Geometry: final body of the model. Coordinates: model frame, mm. Round coordinates to 2 decimals unless told otherwise and drop trailing zeros. Loops run counter-clockwise (first coordinate to the right, second up) from the corner with the lowest first, then second, coordinate; pieces in that order, holes last. Notation, with made-up numbers: (-34.75, -30.5) -> (-14.75, -30.5) arc R15 ccw to (-14.75, -22.5) -> close; hole circle Ø3 at (15, -20). An arc over 180 degrees is marked (long way). Answer in a Markdown table with one row per item.
Autodesk Inventor part; units mm, degrees
ref_plane "YZ Plane" through (0, 0, 0) normal (1, 0, 0) x (0, 1, 0)
ref_plane "XZ Plane" through (0, 0, 0) normal (0, 1, 0) x (-1, 0, 0)
ref_plane "XY Plane" through (0, 0, 0) normal (0, 0, 1) x (1, 0, 0)
sketch "Sketch1" plane through (0, 0, 0) normal (0, 0, 1) x (1, 0, 0)
  line L0 (-75, -15.375) -> (-69, -15.375)
  line L1 (-69, -46.125) -> (-75, -46.125)
  line L2 (-69, 46.125) -> (-75, 46.125)
  line L3 (-75, 15.375) -> (-69, 15.375)
  line L4 (-69, 46.125) -> (-69, 69)
  line L5 (-75, 46.125) -> (-75, 15.375)
  line L6 (-69, 15.375) -> (-69, -15.375)
  line L7 (-75, -15.375) -> (-75, -46.125)
  line L8 (-69, -46.125) -> (-69, -69)
  line L9 (0, 0) -> (0, 15.375)
  line L10 (0, 0) -> (0, -46.125)
  line L11 (69, 15.375) -> (69, -15.375)
  line L12 (75, 15.375) -> (69, 15.375)
  line L13 (75, 46.125) -> (75, 15.375)
  line L14 (69, 46.125) -> (75, 46.125)
  line L15 (69, 46.125) -> (69, 69)
  line L16 (75, -15.375) -> (69, -15.375)
  line L17 (75, -15.375) -> (75, -46.125)
  line L18 (69, -46.125) -> (75, -46.125)
  line L19 (69, -46.125) -> (69, -69)
  line L20 (0, 0) -> (92.4518, 92.4518)
  line L21 (0, 0) -> (102.0745, -102.0745)
  line L22 (-15.375, 75) -> (-15.375, 69)
  line L23 (-46.125, 69) -> (-46.125, 75)
  line L24 (-15.375, 75) -> (-46.125, 75)
  line L25 (-46.125, 69) -> (-69, 69)
  line L26 (15.375, 69) -> (-15.375, 69)
  line L27 (15.375, 75) -> (15.375, 69)
  line L28 (46.125, 75) -> (15.375, 75)
  line L29 (46.125, 69) -> (46.125, 75)
  line L30 (46.125, 69) -> (69, 69)
  line L31 (46.125, -69) -> (46.125, -75)
  line L32 (46.125, -75) -> (15.375, -75)
  line L33 (46.125, -69) -> (69, -69)
  line L34 (-15.375, -75) -> (-15.375, -69)
  line L35 (15.375, -75) -> (15.375, -69)
  line L36 (15.375, -69) -> (-15.375, -69)
  line L37 (-15.375, -75) -> (-46.125, -75)
  line L38 (-46.125, -69) -> (-46.125, -75)
  line L39 (-46.125, -69) -> (-69, -69)
  line L40 (0, 0) -> (-28, 0)
  circle A0 centre (-28, 0) radius 20
  point P0 (0, 0)
  point P1 (0, 0)
  point P2 (-69, -75)
  point P3 (-69, 75)
  point P4 (69, -75)
  point P5 (69, 75)
  dimension "d1" = 28
  dimension "d2" = 40
extrude "Extrusion1" add sketch "Sketch1" along normal blind 6
properties part number "Top"
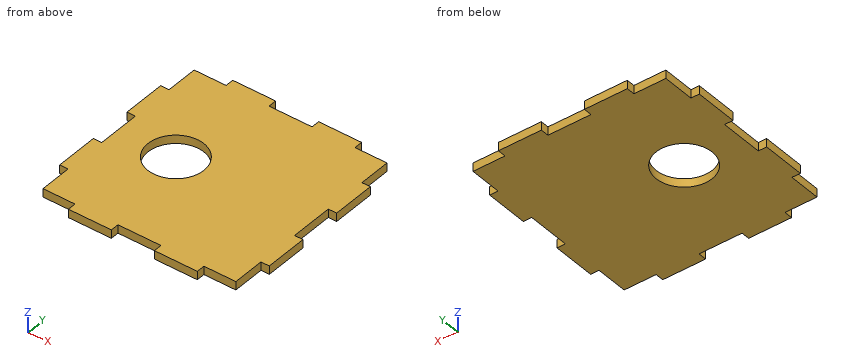
Item 1: Section query A-A, the plane x = -28. Output: boundary loops of the cut face in (y, z), and give its area (3 significant figures).
Ans:
| item | result |
|---|---|
| outline | (-75, 0) -> (-20, 0) -> (-20, 6) -> (-75, 6) -> close; (20, 0) -> (75, 0) -> (75, 6) -> (20, 6) -> close |
| area | 660 mm2 |
Item 2: Section query B-B, the plane y = 0. Output: boundary loops of the cut face in (x, z), and give its area (3 significant figures).
Ans:
| item | result |
|---|---|
| outline | (-69, 0) -> (-48, 0) -> (-48, 6) -> (-69, 6) -> close; (-8, 0) -> (69, 0) -> (69, 6) -> (-8, 6) -> close |
| area | 588 mm2 |
Item 3: First-contact query: P1, Ø1.8, axis at y = -72.5, z = 4.5, coming from the +X side (3 decimals); P2, Ø3, axis at y = -54, z = 3.5, coming from the -X side; P3, Ø1.8, axis at x = -71.5, z = 3, coming from the +Y side (3 decimals). Flat tips, straight axial feed; report the tip coordinate or a pass-through.
Ans:
| item | result |
|---|---|
| P1 | x = 46.125 |
| P2 | x = -69 |
| P3 | y = 46.125 |
Item 4: Ray query, L1, parallel to Y at x = -28, z = 4.4; L2, parallel to Y at x = 2, z = 3.7; L3, parallel to X at y = -12, z = 0.95. Return the intervals inside material, ascending.
Ans:
| item | result |
|---|---|
| L1 | -75 to -20, 20 to 75 |
| L2 | -69 to 69 |
| L3 | -69 to -44, -12 to 69 |
Item 5: Section query C-C, the plane x = -53. Output: boundary loops of the cut face in (y, z), and give its area (3 significant figures).
Ans:
| item | result |
|---|---|
| outline | (-69, 0) -> (69, 0) -> (69, 6) -> (-69, 6) -> close |
| area | 828 mm2 |
